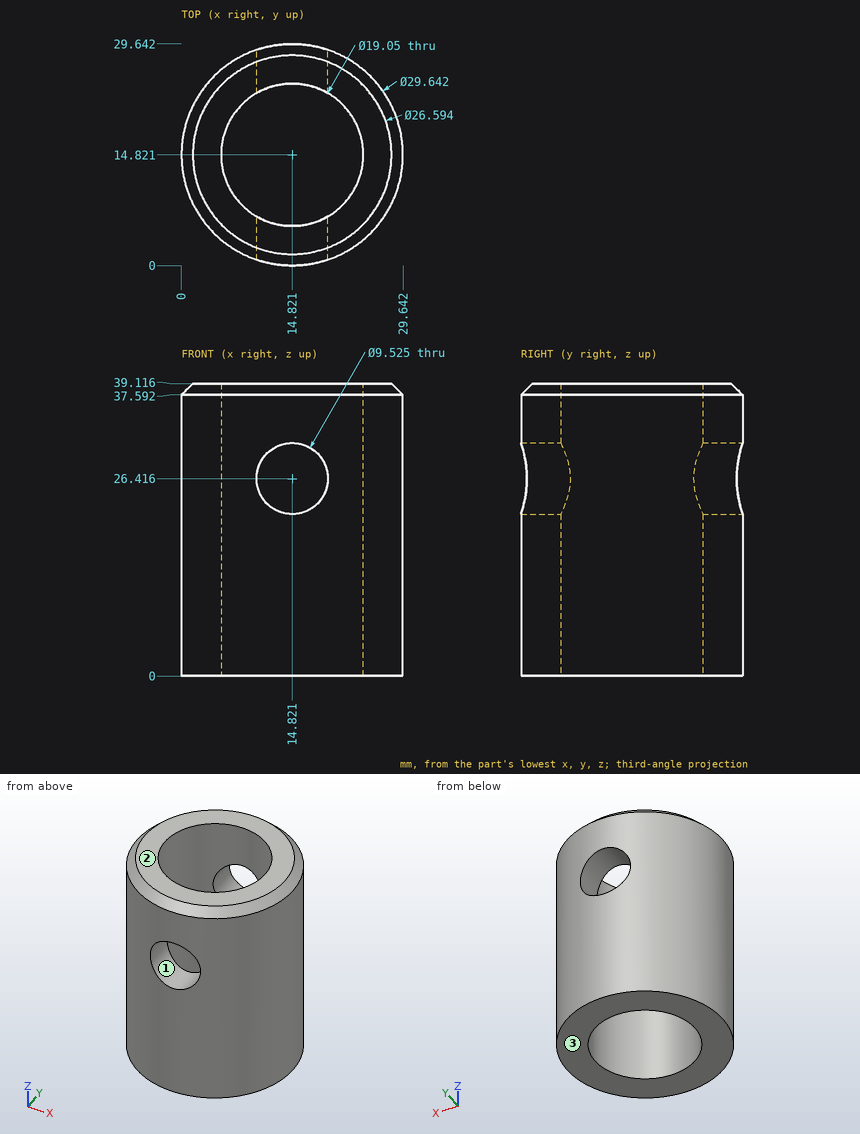
Study the drawing (mm; zero at the part's minimum x, y, z) and answer. Give positions to 0.01 mm unless a question says otherwise; leave off trailing zeros. Return JSON: item names as keys, results as strings. Group by question number.
1. Straight lines are drawn through the part: line 1 (Y direction, x = 20.5, z = 29.5) (1 decimal); line 2 (X direction, y = 9, z = 7); line 3 (X direction, y = 13.25, z = 8.5) (1 decimal). For each, find the intervals that lie inside material, in ascending order. Write a range as [from, to].
2. Given pin 1 Ø10 at (x, z) = (21, 9.5) entering from -Y; pin 2 Ø1 at (x, z) = (15.5, 22) entering from +Y; pin 3 Ø8.5 at (x, z) = (14.82, 26.42) entering from +Y; pin 4 Ø3 at (y, z) = (17.5, 10) entering from +X (3 decimals), each flat-ended and moving along its own axis, determine where each tip first touches the part or whether it passes through.
3. Determine the mould class of the marked faces 1, 2 and 3 for opening direction Z: pulls with the +Z half, pulls with the -Z half, needs draft (parallel to the pull), parting line crosses it, or undercut.
Verdict:
{
 "1": {"line 1": "y = [1.1, 7.2], [22.5, 28.5]", "line 2": "x = [1.19, 7.28], [22.36, 28.45]", "line 3": "x = [0.1, 5.4], [24.2, 29.6]"},
 "2": {"pin 1": "stops at y = 0.05", "pin 2": "stops at y = 29.64", "pin 3": "passes through", "pin 4": "stops at x = 29.595"},
 "3": {"face 1": "undercut", "face 2": "pulls with the +Z half", "face 3": "pulls with the -Z half"}
}
